from build123d import *

# Parameters (mm, degrees)
SKETCH1_W            = 30
SKETCH1_H            = 30.8
BOSS_EXTRUDE1_DEPTH  = 7
SKETCH2_R            = 4.05
CUT_EXTRUDE1_DEPTH   = 6.5
SKETCH3_W            = 15
SKETCH3_H            = 1.2
SKETCH3_W_2          = 9
SKETCH3_W_3          = 11
SKETCH3_W_4          = 13
CUT_EXTRUDE2_DEPTH   = 4
SKETCH4_W            = 30
SKETCH4_H            = 3
CUT_EXTRUDE3_DEPTH   = 1.2
SKETCH5_W            = 30
SKETCH5_H            = 3
CUT_EXTRUDE4_DEPTH   = 1.2
SKETCH6_R            = 4.05
CUT_EXTRUDE5_DEPTH   = 27.2
SKETCH7_R            = 4.05
CUT_EXTRUDE6_DEPTH   = 27.2
SKETCH8_R            = 4.75
CUT_EXTRUDE7_DEPTH   = 5
BOSS_EXTRUDE2_DEPTH  = 6.4
FILLET1_R            = 1
BOSS_EXTRUDE3_DEPTH  = 6.4
FILLET2_R            = 1
SKETCH12_W           = 1.5
SKETCH12_H           = 1.344099237
CUT_EXTRUDE8_DEPTH   = 5
SKETCH13_W           = 13
SKETCH13_H           = 7
BOSS_EXTRUDE4_DEPTH  = 1
SKETCH14_W           = 11
SKETCH14_H           = 7
BOSS_EXTRUDE5_DEPTH  = 1
SKETCH15_R           = 2
BOSS_EXTRUDE8_DEPTH  = 5.5
SKETCH16_R           = 2
BOSS_EXTRUDE9_DEPTH  = 5.5
FILLET3_R            = 2
FILLET4_R            = 2
FILLET5_R            = 2
CHAMFER2_SIZE        = 0.5
CHAMFER3_SIZE        = 0.5
SKETCH17_W           = 4
SKETCH17_H           = 7
BOSS_EXTRUDE10_DEPTH = 1.5
FILLET7_R            = 0.5
SKETCH18_R           = 0.9
CUT_EXTRUDE9_DEPTH   = 99.965895754
SKETCH19_R           = 1.6
CUT_EXTRUDE10_DEPTH  = 2
SKETCH20_R           = 0.9
CUT_EXTRUDE11_DEPTH  = 99.965895754
SKETCH21_R           = 1.6
CUT_EXTRUDE12_DEPTH  = 2
CHAMFER6_SIZE        = 0.5
SKETCH22_W           = 6
SKETCH22_H           = 4
BOSS_EXTRUDE11_DEPTH = 0.5
SKETCH23_W           = 6
SKETCH23_H           = 4
BOSS_EXTRUDE12_DEPTH = 0.5
BOSS_EXTRUDE13_REACH = 100.822
SKETCH24_W           = 4.732966807
SKETCH24_H           = 1.2
SKETCH24_W_2         = 4.75835454


# Some blends are built 0.0001 mm under size
with BuildPart() as part:
    # Sketch1 → Boss-Extrude1 (new body)
    with BuildSketch(Plane(origin=(0, 0, 0), x_dir=(1, 0, 0), z_dir=(0, 1, 0))):
        with Locations((-46.45686042, -50.970505576)):
            Rectangle(SKETCH1_W, SKETCH1_H)
    extrude(amount=BOSS_EXTRUDE1_DEPTH)

    # Sketch2 → Cut-Extrude1 (cut)
    with BuildSketch(Plane.XZ):
        with Locations(Location((-47.47186042, 50.970505576, 0), (0, 0, 270))):
            Circle(SKETCH2_R)
    extrude(amount=-CUT_EXTRUDE1_DEPTH, mode=Mode.SUBTRACT)

    # Sketch3 → Cut-Extrude2 (cut)
    with BuildSketch(Plane.XZ):
        with Locations((-38.95686042, 65.770505576)):
            Rectangle(SKETCH3_W, SKETCH3_H)
        with Locations((-56.95686042, 65.770505576)):
            Rectangle(SKETCH3_W_2, SKETCH3_H)
        with Locations((-36.95686042, 36.170505576)):
            Rectangle(SKETCH3_W_3, SKETCH3_H)
        with Locations((-54.95686042, 36.170505576)):
            Rectangle(SKETCH3_W_4, SKETCH3_H)
    extrude(amount=-CUT_EXTRUDE2_DEPTH, mode=Mode.SUBTRACT)

    # Sketch4 → Cut-Extrude3 (cut)
    with BuildSketch(Plane.XY.offset(66.370505576)):
        with Locations((-46.45686042, 5.5)):
            Rectangle(SKETCH4_W, SKETCH4_H)
    extrude(amount=-CUT_EXTRUDE3_DEPTH, mode=Mode.SUBTRACT)

    # Sketch5 → Cut-Extrude4 (cut)
    with BuildSketch(Plane(origin=(0, 0, 35.570505576), x_dir=(-1, 0, 0), z_dir=(0, 0, -1))):
        with Locations((46.45686042, 5.5)):
            Rectangle(SKETCH5_W, SKETCH5_H)
    extrude(amount=-CUT_EXTRUDE4_DEPTH, mode=Mode.SUBTRACT)

    # Sketch6 → Cut-Extrude5 (cut)
    with BuildSketch(Plane.XY.offset(65.170505576)):
        with Locations((-39.974556342, 7.3)):
            Circle(SKETCH6_R)
    extrude(amount=-CUT_EXTRUDE5_DEPTH, mode=Mode.SUBTRACT)

    # Sketch7 → Cut-Extrude6 (cut)
    with BuildSketch(Plane(origin=(0, 0, 36.770505576), x_dir=(-1, 0, 0), z_dir=(0, 0, -1))):
        with Locations((54.96455223, 7.3)):
            Circle(SKETCH7_R)
    extrude(amount=-CUT_EXTRUDE6_DEPTH, mode=Mode.SUBTRACT)

    # Sketch8 → Cut-Extrude7 (cut)
    with BuildSketch(Plane(origin=(0, 7, 0), x_dir=(1, 0, 0), z_dir=(0, 1, 0))):
        with Locations(Location((-47.47186042, -50.970505576, 0), (0, 0, 270))):
            Circle(SKETCH8_R)
    extrude(amount=-CUT_EXTRUDE7_DEPTH, mode=Mode.SUBTRACT)

    # Sketch10 → Boss-Extrude2 (add)
    with BuildSketch(Plane.XY.offset(65.170505576)):
        Polygon((-31.45686042, 0), (-31.45686042, 7), (-35.85686042, 7), (-35.85686042, 1.7), (-44.45686042, 1.7), (-44.45686042, 0), align=None)
    extrude(amount=BOSS_EXTRUDE2_DEPTH)

    # Fillet1
    fillet1_edges = [part.edges().sort_by_distance(p)[0] for p in [
        (-35.85686042, 1.7, 68.370505576),
    ]]
    fillet(fillet1_edges, radius=FILLET1_R)

    # Sketch11 → Boss-Extrude3 (add)
    with BuildSketch(Plane(origin=(0, 0, 36.770505576), x_dir=(-1, 0, 0), z_dir=(0, 0, -1))):
        Polygon((61.45686042, 7), (61.45686042, 0), (50.45686042, 0), (50.45686042, 1.7), (59.05686042, 1.7), (59.05686042, 7), align=None)
    extrude(amount=BOSS_EXTRUDE3_DEPTH)

    # Fillet2
    fillet2_edges = [part.edges().sort_by_distance(p)[0] for p in [
        (-59.05686042, 1.7, 33.570505576),
    ]]
    fillet(fillet2_edges, radius=FILLET2_R)

    # Sketch12 → Cut-Extrude8 (cut)
    with BuildSketch(Plane(origin=(0, 7, 0), x_dir=(1, 0, 0), z_dir=(0, 1, 0))):
        with Locations((-47.47186042, -56.298455958)):
            Rectangle(SKETCH12_W, SKETCH12_H)
    extrude(amount=-CUT_EXTRUDE8_DEPTH, mode=Mode.SUBTRACT)

    # Sketch13 → Boss-Extrude4 (add)
    with BuildSketch(Plane.XY.offset(71.570505576)):
        with Locations((-37.95686042, 3.5)):
            Rectangle(SKETCH13_W, SKETCH13_H)
    extrude(amount=BOSS_EXTRUDE4_DEPTH)

    # Sketch14 → Boss-Extrude5 (add)
    with BuildSketch(Plane(origin=(0, 0, 30.370505576), x_dir=(-1, 0, 0), z_dir=(0, 0, -1))):
        with Locations((55.95686042, 3.5)):
            Rectangle(SKETCH14_W, SKETCH14_H)
    extrude(amount=BOSS_EXTRUDE5_DEPTH)

    # Sketch15 → Boss-Extrude8 (add)
    with BuildSketch(Plane.XY.offset(71.570505576)):
        with Locations(Location((-36.96455223, 6.8, 0), (0, 0, 174.260829523))):
            Circle(SKETCH15_R)
    extrude(amount=BOSS_EXTRUDE8_DEPTH)

    # Sketch16 → Boss-Extrude9 (add)
    with BuildSketch(Plane(origin=(0, 0, 30.370505576), x_dir=(-1, 0, 0), z_dir=(0, 0, -1))):
        with Locations(Location((57.974556342, 6.8, 0), (0, 0, 174.260829523))):
            Circle(SKETCH16_R)
    extrude(amount=BOSS_EXTRUDE9_DEPTH)

    # Fillet3
    fillet3_edges = [part.edges().sort_by_distance(p)[0] for p in [
        (-59.964531217, 7, 29.870505576),
    ]]
    fillet(fillet3_edges, radius=FILLET3_R)

    # Fillet4
    # the kernel refuses this fillet: 2 mm, written as the material it adds along each edge
    with BuildSketch(Plane(origin=(-55.984581468, 7, 30.370505576), x_dir=(1.0, 7.52728269616064e-12, 0), z_dir=(0, 0, -1))) as fillet4_piece_1:
        with BuildLine():
            CenterArc((1.350683743, -2), FILLET4_R, 90, 56.632987031)
            ThreePointArc((-0.319645565, -0.9), (-0.105311329, -0.469360383), (0, 0))
            Line((0, 0), (1.350683743, 0))
        make_face()
    extrude(amount=1)

    # Fillet5
    # the kernel refuses this fillet: 2 mm, written as the material it adds along each edge
    with BuildSketch(Plane(origin=(-38.954527104, 7, 71.570505576), x_dir=(-1.0, 7.116297137925098e-12, 0), z_dir=(0, 0, 1)), Plane(origin=(-34.974577356, 7, 72.570505576), x_dir=(1, 0, 0), z_dir=(0, 0, -1))) as fillet5_piece_1:
        with BuildLine():
            CenterArc((1.350683743, -2), FILLET5_R, 90, 56.632987031)
            ThreePointArc((-0.319645565, -0.9), (-0.105311329, -0.469360383), (0, 0))
            Line((0, 0), (1.350683743, 0))
        make_face()
    extrude(amount=1)

    # Chamfer2
    chamfer2_edges = [part.edges().sort_by_distance(p)[0] for p in [
        (-34.974577356, 6.6, 77.070505576),
    ]]
    chamfer(chamfer2_edges, length=CHAMFER2_SIZE)

    # Chamfer3
    chamfer3_edges = [part.edges().sort_by_distance(p)[0] for p in [
        (-59.964531217, 6.6, 24.870505576),
    ]]
    chamfer(chamfer3_edges, length=CHAMFER3_SIZE)

    # Sketch17 → Boss-Extrude10 (add)
    with BuildSketch(Plane(origin=(-31.45686042, 0, 0), x_dir=(0, 0, -1), z_dir=(1, 0, 0))):
        with Locations((-50.970505576, 3.5)):
            Rectangle(SKETCH17_W, SKETCH17_H)
    extrude(amount=BOSS_EXTRUDE10_DEPTH)

    # Fillet7
    fillet7_edges = [part.edges().sort_by_distance(p)[0] for p in [
        (-31.45686042, 3.5, 52.970505576),
        (-31.45686042, 3.5, 48.970505576),
        (-29.95686042, 3.5, 52.970505576),
        (-29.95686042, 3.5, 48.970505576),
    ]]
    fillet(fillet7_edges, radius=FILLET7_R)

    # Sketch18 → Cut-Extrude9 (cut, through all)
    with BuildSketch(Plane.XZ):
        with Locations(Location((-32.45686042, 50.970505576, 0), (0, 0, 270))):
            Circle(SKETCH18_R)
    extrude(amount=-CUT_EXTRUDE9_DEPTH, mode=Mode.SUBTRACT)

    # Sketch19 → Cut-Extrude10 (cut)
    with BuildSketch(Plane.XZ):
        with Locations(Location((-32.45686042, 50.970505576, 0), (0, 0, 270))):
            Circle(SKETCH19_R)
    extrude(amount=-CUT_EXTRUDE10_DEPTH, mode=Mode.SUBTRACT)

    # Sketch20 → Cut-Extrude11 (cut, through all)
    with BuildSketch(Plane.XZ):
        with Locations(Location((-47.45686042, 62.720505576, 0), (0, 0, 270))):
            Circle(SKETCH20_R)
        with Locations(Location((-47.45686042, 39.220505576, 0), (0, 0, 270))):
            Circle(SKETCH20_R)
    extrude(amount=-CUT_EXTRUDE11_DEPTH, mode=Mode.SUBTRACT)

    # Sketch21 → Cut-Extrude12 (cut)
    with BuildSketch(Plane.XZ):
        with Locations(Location((-47.45686042, 62.720505576, 0), (0, 0, 270))):
            Circle(SKETCH21_R)
        with Locations(Location((-47.45686042, 39.220505576, 0), (0, 0, 270))):
            Circle(SKETCH21_R)
    extrude(amount=-CUT_EXTRUDE12_DEPTH, mode=Mode.SUBTRACT)

    # Chamfer6
    chamfer6_edges = [part.edges().sort_by_distance(p)[0] for p in [
        (-61.45686042, 0, 47.270505576),
        (-31.45686042, 0, 63.020505576),
        (-30.70686042, 0, 52.970505576),
        (-29.95686042, 0, 50.970505576),
        (-31.45686042, 0, 42.620505576),
        (-30.70686042, 0, 48.970505576),
        (-30.103307029, 0, 49.116952185),
        (-30.103307029, 0, 52.824058967),
        (-31.310413811, 0, 53.116952185),
        (-31.310413811, 0, 48.824058967),
    ]]
    chamfer(chamfer6_edges, length=CHAMFER6_SIZE - 0.0001)  # a hair under: the kernel refuses the full size

    # Sketch22 → Boss-Extrude11 (add)
    with BuildSketch(Plane(origin=(0, 0, 35.570505576), x_dir=(-1, 0, 0), z_dir=(0, 0, -1))):
        with Locations((45.45686042, 2)):
            Rectangle(SKETCH22_W, SKETCH22_H)
    extrude(amount=BOSS_EXTRUDE11_DEPTH)

    # Sketch23 → Boss-Extrude12 (add)
    with BuildSketch(Plane.XY.offset(66.370505576)):
        with Locations((-49.45686042, 2)):
            Rectangle(SKETCH23_W, SKETCH23_H)
    extrude(amount=BOSS_EXTRUDE12_DEPTH)

    # Boss-Extrude13: up to this face of the body (flat: up to its plane)
    boss_extrude13_end = Plane(part.part.faces().sort_by_distance((-54.25686042, 1.7, 33.570505576))[0])
    # Sketch24 → Boss-Extrude13 (add, up to the picked face)
    with BuildSketch(Plane(origin=(0, 7, 0), x_dir=(1, 0, 0), z_dir=(0, 1, 0)), mode=Mode.PRIVATE) as boss_extrude13_sk1:
        with Locations((-35.990377017, -70.970505576)):
            Rectangle(SKETCH24_W, SKETCH24_H)
    boss_extrude13_tool1 = split(extrude(boss_extrude13_sk1.sketch, amount=-BOSS_EXTRUDE13_REACH, mode=Mode.PRIVATE), bisect_by=boss_extrude13_end, keep=Keep.BOTH, mode=Mode.PRIVATE)
    # Sketch24 → Boss-Extrude13 (add, up to the picked face)
    with BuildSketch(Plane(origin=(0, 7, 0), x_dir=(1, 0, 0), z_dir=(0, 1, 0)), mode=Mode.PRIVATE) as boss_extrude13_sk2:
        with Locations((-58.93603769, -30.970505576)):
            Rectangle(SKETCH24_W_2, SKETCH24_H)
    boss_extrude13_tool2 = split(extrude(boss_extrude13_sk2.sketch, amount=-BOSS_EXTRUDE13_REACH, mode=Mode.PRIVATE), bisect_by=boss_extrude13_end, keep=Keep.BOTH, mode=Mode.PRIVATE)
    add(boss_extrude13_tool1.solids().sort_by(Axis((-35.990377, 7, 70.970506), (0, -1, 0)))[0])
    add(boss_extrude13_tool2.solids().sort_by(Axis((-58.936038, 7, 30.970506), (0, -1, 0)))[0])


solid = part.part
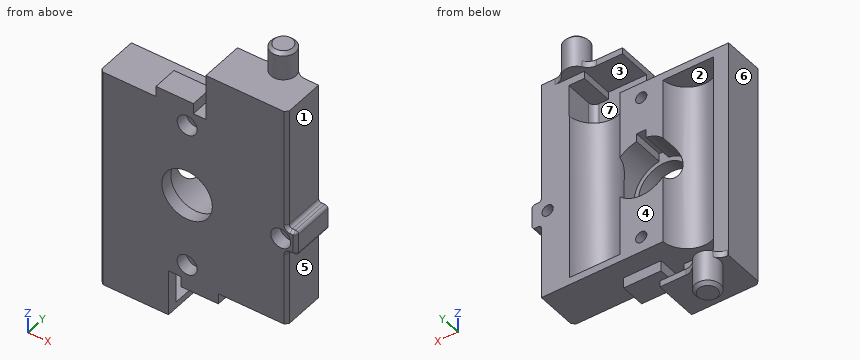
Input: part model. Units: mm. Frame: model coordinates. Face numbers are marked on the shaded views. A direction names the side the tool comes from. Coordinates: 2 decimals unless noted, no trailing zeros.
1. Draft query along X for the marked faces 4, 5, 6 and 7. Return one class per face: +X half, -X half, draft (parallel to the pull), parting line (faces both ways), or undercut.
Checked values:
face 4: draft
face 5: +X half
face 6: -X half
face 7: undercut
2. Ray query, line 1 along Z through (x, y) = (-47, 1.25); line 2 along X through (y, z) = (4.5, 62); line 3 along Z through (x, y) = (-45, 2.75). Return the intervals inside material, ascending.
Checked values:
line 1: z = 35.07 to 37.69, 40.75 to 46.95, 54.99 to 61.19, 64.25 to 66.87
line 2: x = -61.46 to -57.89, -52.04 to -48, -46.92 to -42.9, -37.05 to -31.46
line 3: z = 35.07 to 46.91, 55.03 to 65.17
3. Access query for the marked faces 1, 2 and 3. Directions: +Z, -Z, +X, -X, +Y, -Y. A direction counts if a zero-diameter tool reaches every point of the face in a straight line with its end or side. Return the directions, or none.
Checked values:
face 1: +Z, +X, +Y, -Y
face 2: +Y
face 3: -X, +Y
4. Contact query for flat-ended pins moving along their axis: P1, Ø1.4, axis at x = -50, z = 66, coming from the +Y side; P2, Ø6, axis at x = -37, z = 42.5, coming from the +Y side; P3, Ø4, axis at y = 8, z = 65.5, coming from the +X side. Output: stop coordinate, or through.
Checked values:
P1: stops at y = 4
P2: stops at y = 7
P3: stops at x = -31.46
